from build123d import *

# Parameters (mm, degrees)
F0_W          = 12
F0_H          = 14.76
F1_DEPTH      = 1
F3_DEPTH      = 25.4
F3_DEPTH_BACK = 25.4
F4_SIZE2      = 0.9330127019
F4_SIZE       = 0.25


with BuildPart() as f1:
    # F0 (on Top) → F1 (new body)
    with BuildSketch(Plane.XY):
        Rectangle(F0_W, F0_H)
    extrude(amount=F1_DEPTH)

    # F2 (on face) → F3 (cut, two sides)
    with BuildSketch(Plane.XY.offset(1)) as f3_sk:
        with BuildLine():
            ThreePointArc((-6, 7.38), (0, 1.38), (6, 7.38))
            Line((6, 7.38), (-6, 7.38))
        make_face()
    extrude(amount=-F3_DEPTH, mode=Mode.SUBTRACT)
    extrude(f3_sk.sketch, amount=F3_DEPTH_BACK, mode=Mode.SUBTRACT)

    # F4
    f4_edges = [f1.edges().sort_by_distance(p)[0] for p in [
        (0, 1.38, 0),
    ]]
    f4_side = f1.faces().sort_by_distance((0, -2.26695, 0))[0]
    chamfer(f4_edges, length=F4_SIZE, length2=F4_SIZE2, reference=f4_side)


solid = f1.part
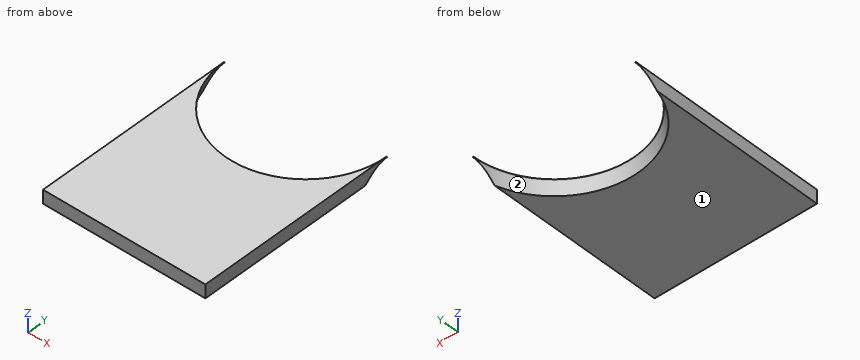
Design review of the part built by this model. Coordinates are the model's own, in mm. Face numbers are marked on the shaded views. Coordinates: 2 decimals unless noted, no trailing zeros. Order: outer loops, then holes, each group sorted by start corner. A loop starts at its lowest first (then second) coordinate and runs counter-clockwise, first axis right, second up. Notation, with made-up numbers: M 65.25,57.5 L 98.25,57.5 A15 cw 98.25,63.5 Z; hole C -18.5,12 d3. An arc over 180 degrees is marked long. Use a Markdown table: item, result.
(1) Draft analysis for pull direction X (two halves, no side actions). For the marked faces 1 and 2, state which applies: released by +X, released by -X, zero draft, split by the parting line, or undercut.
Worked answers:
| item | result |
|---|---|
| face 1 | zero draft |
| face 2 | undercut |
(2) Wall thickness on probe 1 along X at (y, z) = (2, 0.75); probe 2 along X at (y, z) = (5, 0.1); probe 3 along Y at (x, z) = (-4.5, 0.65): over which ranges is each line inside the solid? List them lowest first.
Worked answers:
| item | result |
|---|---|
| probe 1 | x = -6 to -2.77, 2.77 to 6 |
| probe 2 | x = -6 to -5.75, 5.75 to 6 |
| probe 3 | y = -7.38 to 3.3 |
(3) Add section A-A (x = 0). Give the boundary of the cut face in (y, z).
Worked answers:
| item | result |
|---|---|
| outline | M -7.38,0 L 1.13,0 L 1.38,0.93 L 1.38,1 L -7.38,1 Z |
(4) Add section B-B (z = 0.4). Give the boundary of the cut face in (x, y).
Worked answers:
| item | result |
|---|---|
| outline | M -6,-7.38 L 6,-7.38 L 6,6.06 A6.14 cw -6,6.06 Z |
